CAD build for the part. Positions are in the model's coordinates, mm. Face numbers are marked on the shaded views. A direction names the side the tool comes from. Coordinates: 2 decimals unless noted, no trailing zeros. Loops run counter-clockwise (first coordinate to the right, second up) from the corner with the lowest first, then second, coordinate; pieces in that order, holes last. Notation, with made-up numbers: (8, 4) -> (20, 4) arc R18 ccw to (20, 33) -> close; hole circle Ø4 at (74.25, -15.75). An arc over 180 degrees is marked (long way). Return JSON: item names as keys, results as strings. Group by question number.
(1) Saw through at A-A on x = 0. Give the number of separate pieces and of enclosed holes in the cut face, then the cut area to 3 significant figures.
(2) Mould opens along Y. For the marked faces 3, 4, 5 and 6 say: pulls with the +Y half, pulls with the -Y half, needs draft (parallel to the pull), parting line crosses it, or undercut.
(3) Tool access for the marked faces 1 and 2: list every direction of +Z, -Z, +X, -X, +Y, -Y with a clear straight run to the whole face (end or side of a thin tool).
(4) Probe L1, parallel to Y at x = 7.5, z = 6.25; L2, parallel to X at y = 21.1, z = 0; L3, parallel to Y at x = 8.25, z = 0.75. List the from-to ranges inside material, lowest first.
(5) Saw through at D-D on y = 1.75. Write the cut outline in (x, z).
(6) Saw through at B-B on y = 4. Write the cut outline in (x, z), then the cut area to 3 significant figures.
(7) Flat gauge pins, fed straight in: pin 1 Ø10 at (y, z) = (4, 5.5) entering from +X; pin 2 Ø8 at (y, z) = (17.5, -3.5) entering from -X; pin 3 Ø8 at (x, y) = (1, 14) entering from +Z; pin 4 Ø1.5 at (y, z) = (19, 7.5) entering from -X (3 decimals). Where does each tip first touch, or does it go through?
(8) Saw through at C-C on y = 20.75. Write the cut outline in (x, z).
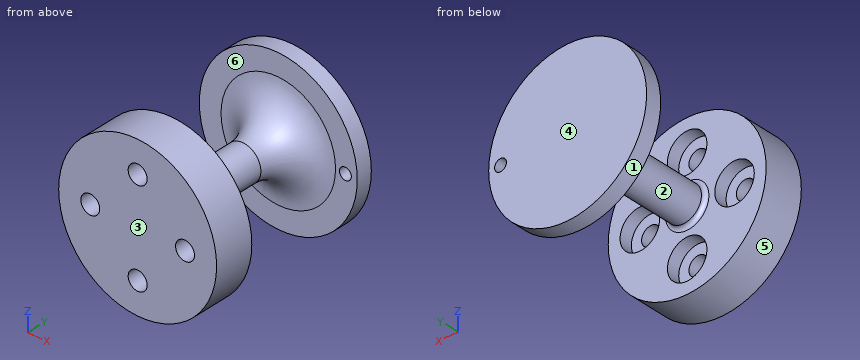
```python
from build123d import *

# Parameters (mm, degrees)
SKETCH1_R                                = 10
BOTTOM_DEPTH                             = 5
CBORE_FOR_M2_PAN_HEAD_SCREW1_D           = 2.4
CBORE_FOR_M2_PAN_HEAD_SCREW1_CBORE_D     = 5
CBORE_FOR_M2_PAN_HEAD_SCREW1_CBORE_DEPTH = 1.6
SKETCH4_R                                = 2.25
GROOVE_DEPTH                             = 15
CIRPATTERN1_COUNT                        = 4
FILLET1_R                                = 0.5
SKETCH7_R                                = 10
TOP_DEPTH                                = 2
SKETCH8_R                                = 0.75
THREAD_TERMINAL_DEPTH                    = 2
FILLET2_R                                = 5


with BuildPart() as part:
    # Sketch1 → bottom (new body)
    with BuildSketch(Plane(origin=(0, 0, 0), x_dir=(1, 0, 0), z_dir=(0, 1, 0))):
        with Locations(Location((0, 0, 0), (0, 0, 270))):
            Circle(SKETCH1_R)
    extrude(amount=BOTTOM_DEPTH)

    # CBORE for M2 Pan Head Screw1 (through all)
    with Locations(Plane(origin=(0, 5, 0), x_dir=(1, 0, 0), z_dir=(0, 1, 0))):
        with Locations((6, 0)):
            cbore_for_m2_pan_head_screw1 = CounterBoreHole(CBORE_FOR_M2_PAN_HEAD_SCREW1_D / 2, CBORE_FOR_M2_PAN_HEAD_SCREW1_CBORE_D / 2, CBORE_FOR_M2_PAN_HEAD_SCREW1_CBORE_DEPTH)

    # Sketch4 → groove (add)
    with BuildSketch(Plane(origin=(0, 5, 0), x_dir=(1, 0, 0), z_dir=(0, 1, 0))):
        with Locations(Location((0, 0, 0), (0, 0, 270))):
            Circle(SKETCH4_R)
    extrude(amount=GROOVE_DEPTH)

    # CirPattern1: CBORE for M2 Pan Head Screw1 ×4 about axis
    cirpattern1_axis = Axis((0, 0, 0), (0, 1, 0))
    for i in range(1, CIRPATTERN1_COUNT):
        add(cbore_for_m2_pan_head_screw1.rotate(cirpattern1_axis, i * 360 / CIRPATTERN1_COUNT), mode=Mode.SUBTRACT)

    # Fillet1
    fillet1_edges = [part.edges().sort_by_distance(p)[0] for p in [
        (0, 5, -2.25),
    ]]
    fillet(fillet1_edges, radius=FILLET1_R)

    # Sketch7 → top (add)
    with BuildSketch(Plane(origin=(0, 20, 0), x_dir=(1, 0, 0), z_dir=(0, 1, 0))):
        with Locations(Location((0, 0, 0), (0, 0, 270))):
            Circle(SKETCH7_R)
    extrude(amount=TOP_DEPTH)

    # Sketch8 → thread_terminal (cut)
    with BuildSketch(Plane(origin=(0, 22, 0), x_dir=(1, 0, 0), z_dir=(0, 1, 0))):
        with Locations(Location((8.5, 0, 0), (0, 0, 270))):
            Circle(SKETCH8_R)
    extrude(amount=-THREAD_TERMINAL_DEPTH, mode=Mode.SUBTRACT)

    # Fillet2
    fillet2_edges = [part.edges().sort_by_distance(p)[0] for p in [
        (0, 20, -2.25),
    ]]
    fillet(fillet2_edges, radius=FILLET2_R)


solid = part.part
```
Geometry results:
{
 "1": {"separate pieces": "3", "enclosed holes": "0", "area": "186 mm²"},
 "2": {"face 3": "pulls with the -Y half", "face 4": "pulls with the +Y half", "face 5": "needs draft", "face 6": "undercut"},
 "3": {"face 1": "+Y, -Y", "face 2": "none"},
 "4": {"L1": "0 to 5, 20 to 22", "L2": "-10 to 7.75, 9.25 to 10", "L3": "0 to 3.4, 20 to 22"},
 "5": {"outline": "circle Ø20 at (0, 0); hole circle Ø2.4 at (-6, 0); hole circle Ø2.4 at (0, -6); hole circle Ø2.4 at (0, 6); hole circle Ø2.4 at (6, 0)"},
 "6": {"outline": "circle Ø20 at (0, 0); hole circle Ø5 at (-6, 0); hole circle Ø5 at (0, -6); hole circle Ø5 at (0, 6); hole circle Ø5 at (6, 0)", "area": "236 mm²"},
 "7": {"pin 1": "x = 9.99", "pin 2": "x = -9.99", "pin 3": "z = 3.19", "pin 4": "through"},
 "8": {"outline": "circle Ø20 at (0, 0); hole circle Ø1.5 at (8.5, 0)"}
}
